```python
from build123d import *

# Parameters (mm, degrees)
CHANFREIN1_SIZE         = 0.6905
CHANFREIN1_SIZE2        = 0.398660361
ESQUISSE3_R             = 2.55
ENL_V_MAT_EXTRU_2_DEPTH = 2.2
ESQUISSE4_R             = 4
ENL_V_MAT_EXTRU_3_DEPTH = 12.2
CHANFREIN2_SIZE         = 0.6
ESQUISSE5_OUTSIDE_W     = 12.772
ESQUISSE5_OUTSIDE_H     = 12.772
ESQUISSE5_OUTSIDE_R     = 3.7
ENL_V_MAT_EXTRU_4_DEPTH = 10.797958971
ESQUISSE6_W             = 1
ESQUISSE6_H             = 2.203007131
ENL_V_MAT_EXTRU_5_DEPTH = 2
ESQUISSE7_R             = 1
ENL_V_MAT_EXTRU_6_DEPTH = 8.81152994


with BuildPart() as part:
    # Esquisse1 → Révolution1 (revolve)
    with BuildSketch(Plane.XY, mode=Mode.PRIVATE) as r_volution1_sk:
        Polygon((0, 4), (0, 0), (12.000000001, 0), (8, 4), align=None)
    revolve(r_volution1_sk.sketch.rotate(Axis((0, 0, 0), (1, 0, 0)), 270), axis=Axis((0, 0, 0), (1, 0, 0)))

    # Chanfrein1
    chanfrein1_edges = [part.edges().sort_by_distance(p)[0] for p in [
        (0, 0, 4),
    ]]
    chanfrein1_side = [part.faces().sort_by_distance(p)[0] for p in [
        (0, 0, 0),
    ]]
    chamfer(chanfrein1_edges, length=CHANFREIN1_SIZE, length2=CHANFREIN1_SIZE2, reference=chanfrein1_side[0])

    # Esquisse3 → Enlèv. mat.-Extru.2 (cut)
    with BuildSketch(Plane.ZY):
        Circle(ESQUISSE3_R)
    extrude(amount=-ENL_V_MAT_EXTRU_2_DEPTH, mode=Mode.SUBTRACT)

    # Esquisse4 → Enlèv. mat.-Extru.3 (cut)
    with BuildSketch(Plane.ZY.offset(-8)):
        Circle(ESQUISSE4_R)
    extrude(amount=-ENL_V_MAT_EXTRU_3_DEPTH, mode=Mode.SUBTRACT)

    # Chanfrein2
    chanfrein2_edges = [part.edges().sort_by_distance(p)[0] for p in [
        (8, 0, 4),
    ]]
    chamfer(chanfrein2_edges, length=CHANFREIN2_SIZE)

    # Esquisse5 outside → Enlèv. mat.-Extru.4 (cut, through all)
    with BuildSketch(Plane.ZY):
        Rectangle(ESQUISSE5_OUTSIDE_W, ESQUISSE5_OUTSIDE_H)
        Circle(ESQUISSE5_OUTSIDE_R, mode=Mode.SUBTRACT)
    extrude(amount=-ENL_V_MAT_EXTRU_4_DEPTH, mode=Mode.SUBTRACT)

    # Esquisse6 → Enlèv. mat.-Extru.5 (cut)
    with BuildSketch(Plane.ZY):
        with Locations((0, 3.309500001)):
            Rectangle(ESQUISSE6_W, ESQUISSE6_H)
    extrude(amount=-ENL_V_MAT_EXTRU_5_DEPTH, mode=Mode.SUBTRACT)

    # Esquisse7 → Enlèv. mat.-Extru.6 (cut, through all)
    with BuildSketch(Plane.ZY.offset(-2.2)):
        Circle(ESQUISSE7_R)
    extrude(amount=-ENL_V_MAT_EXTRU_6_DEPTH, mode=Mode.SUBTRACT)


solid = part.part
```
Could you check a few things on this model? Use its own coordinates, in mm. A direction names the side the tool comes from. Give positions to 0.01 mm unless a question says otherwise; leave off trailing zeros. Loops run counter-clockwise (first coordinate to the right, second up) from the corner with the lowest first, then second, coordinate; pieces in that order, holes last. Notation, with made-up numbers: (45.25, -39.5) -> (69.25, -39.5) arc R15 ccw to (69.25, -25.5) -> close; hole circle Ø9 at (62.25, 77.5). An arc over 180 degrees is marked (long way). Put each result on its own line as item: value.
(1) Please list where these lines run through material, in increasing order: probe 1 along Z at (x, y) = (1.3, 0); probe 2 along Y at (x, z) = (4.95, 0); probe 3 along Z at (x, y) = (0.5, 1.25). Write a range as [from, to].
Computed:
probe 1: [-3.7, -2.55], [2.55, 3.7]
probe 2: [-3.7, -1], [1, 3.7]
probe 3: [-3.48, -2.22], [2.22, 3.48]
(2) Imagine slicing it at D-D on x = 1.25. Write out the boundary of the cut face in (y, z).
Computed:
outline: (2.5, -0.5) arc R2.55 cw (long way) to (2.5, 0.5) -> (3.67, 0.5) arc R3.7 ccw (long way) to (3.67, -0.5) -> close
(3) Thinking about a two-plate mould opening in Y: for faces 4 (the face through (5, -1, 0)), 5 (the face through (1.08, -2.26, 1.18)), 6 (the face through (1, 3, 0.5)), 7 (the face through (3.91, -3.612, -0.802)), which applies, pulls with the +Y half, pulls with the -Y half, needs draft (parallel to the pull), parting line crosses it, or undercut?
Computed:
face 4: undercut
face 5: undercut
face 6: needs draft
face 7: parting line crosses it
(4) Imagine slicing it at C-C on x = 2.75. Write out the boundary of the cut face in (y, z).
Computed:
outline: circle Ø7.4 at (0, 0); hole circle Ø2 at (0, 0)
(5) Imagine slicing it at A-A on y = 0. Write out the boundary of the cut face in (x, z).
Computed:
outline: (0, -3.31) -> (0.23, -3.7) -> (7.7, -3.7) -> (8, -3.4) -> (8, -1) -> (2.2, -1) -> (2.2, -2.55) -> (0, -2.55) -> close; (0, 2.55) -> (2.2, 2.55) -> (2.2, 1) -> (8, 1) -> (8, 3.4) -> (7.7, 3.7) -> (0.23, 3.7) -> (0, 3.31) -> close
(6) I'm going to push flat-ended pins straight in: pin 1 Ø4 at (x, z) = (7, -2.5) entering from +Y; pin 2 Ø3 at (y, z) = (0, 0) entering from +X; pin 3 Ø3 at (y, z) = (0, 0) entering from -X; pin 4 Ø0.5 at (y, z) = (3, 0) entering from -X. Where does each tip first touch, or does it pass through?
Computed:
pin 1: y = 3.67
pin 2: x = 8
pin 3: x = 2.2
pin 4: x = 2
(7) Imagine slicing it at B-B on z = 0. Write out the boundary of the cut face in (x, y).
Computed:
outline: (0, -3.31) -> (0.23, -3.7) -> (7.7, -3.7) -> (8, -3.4) -> (8, -1) -> (2.2, -1) -> (2.2, -2.55) -> (0, -2.55) -> close; (2, 2.55) -> (2.2, 2.55) -> (2.2, 1) -> (8, 1) -> (8, 3.4) -> (7.7, 3.7) -> (2, 3.7) -> close
(8) For faces 1 (the face through (0, -2, -2)), 2 (the face through (2.2, -1, 1)), 3 (the face through (2, 3, 0)), which set-ups out of +Z, -Z, +X, -X, +Y, -Y let a thin tool reach every point of the face, with its end or its side?
Computed:
face 1: +Z, -Z, -X, +Y, -Y
face 2: -X
face 3: -X, +Y
